Drawing for the job (mm, zero at the part's lowest x, y, z). A direction names the side the tool comes from. Round coordinates to 2 decimals unless told otherwise and drop trailing zeros. Order: outer loops, then holes, each group sorted by start corner. A loop starts at its lowest first (then second) coordinate and runs counter-clockwise, first axis right, second up. Notation, with made-up numbers: (71.25, -27) - (79.25, -27) arc R20 cw to (79.25, 10) - close; hole circle Ø7 at (4.25, 41). An arc over 180 degrees is marked (long way). Answer as a JSON object with one key per item and string values.
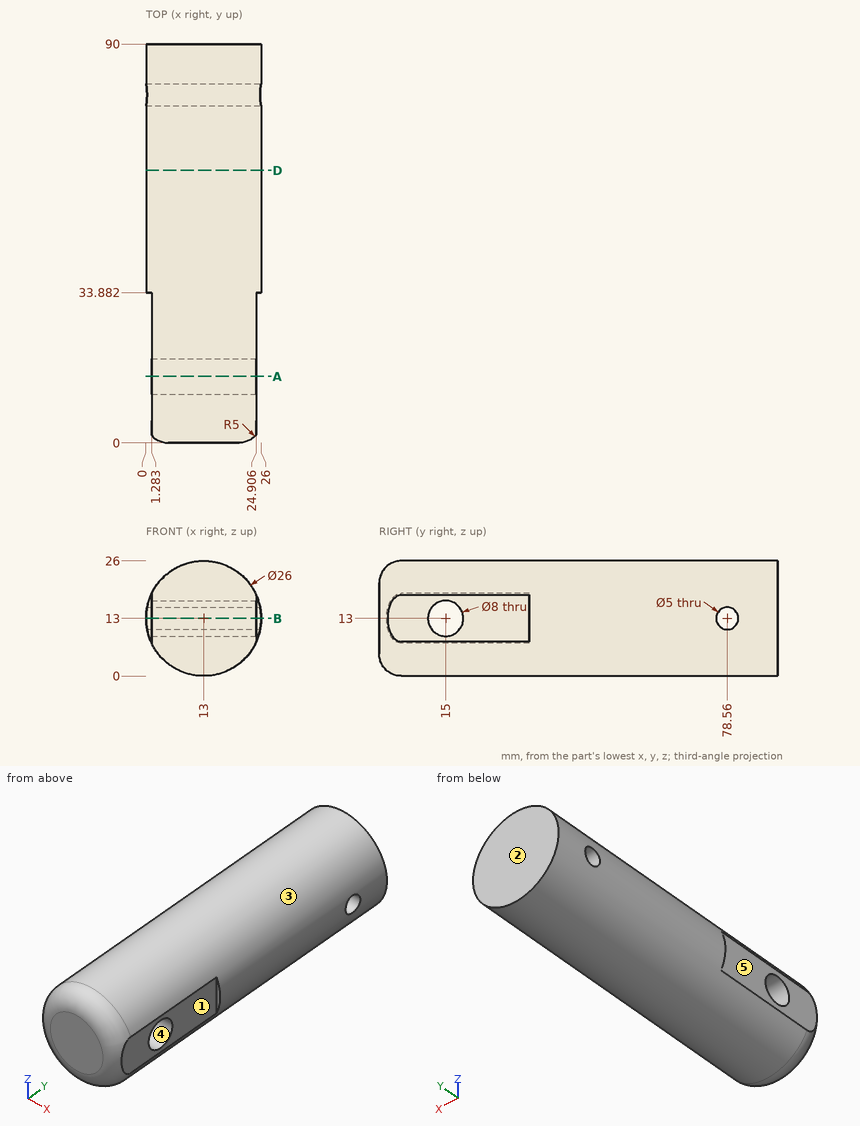
Item 1: Two-plate mould, pull along Z, no slides. Class the marked faces 3, 4 and 5: pulls with the +Z half, pulls with the -Z half, needs draft (parallel to the pull), parting line crosses it, or undercut.
Taken from the geometry:
{"face 3": "parting line crosses it", "face 4": "undercut", "face 5": "needs draft"}
Item 2: Drop flat-ended pins along their axis: P1, Ø3.5, axis at y = 17, z = 15.5, coming from the -X side; P2, Ø6, axis at y = 78.56, z = 13, coming from the -X side; P3, Ø4, axis at x = 20, y = 33.5, coming from the +Z side; P4, Ø1, axis at x = 5.5, y = 50, coming from the -Z side (1 decimal). Give the stop position or say it passes through.
Taken from the geometry:
{"P1": "x = 1.28", "P2": "x = 0", "P3": "z = 25", "P4": "z = 2"}
Item 3: Cut at A-A (y = 15). Write the cut outline in (x, z).
Taken from the geometry:
{"outline": "(1.28, 7.37) arc R13 ccw to (24.91, 7.78) - (24.91, 9) - (1.28, 9) - close; (1.28, 17) - (24.91, 17) - (24.91, 18.22) arc R13 ccw to (1.28, 18.63) - close"}
Item 4: Cut at B-B (z = 13). State how many separate pieces and enclosed holes the cut face has, plus the area to 3 significant figures.
Taken from the geometry:
{"separate pieces": "3", "enclosed holes": "0", "area": "1,940 mm2"}
Item 5: Probe L1, parallel to Y at x = 17.25, z = 13; L2, parallel to Y at x = 16.5, z = 11.75 (1 decimal); L3, parallel to X at y = 67, z = 13.5. List the from-to ranges inside material, lowest first. Write a range as from..to.
Taken from the geometry:
{"L1": "0..11, 19..76.06, 81.06..90", "L2": "0..11.2, 18.8..76.4, 80.7..90", "L3": "0.01..25.99"}
Item 6: Cut at D-D (y = 61.5). Write the cut outline in (x, z), plus the area to 3 significant figures.
Taken from the geometry:
{"outline": "circle Ø26 at (13, 13)", "area": "531 mm2"}
Item 7: Tool access for the marked faces 1 and 2: list every direction of +Z, -Z, +X, -X, +Y, -Y with a clear straight run to the whole face (end or side of a thin tool).
Taken from the geometry:
{"face 1": "+Z, -Z, +X, -Y", "face 2": "+Z, -Z, +X, -X, +Y"}
